from build123d import *

# Parameters (mm, degrees)
REVOLUTION002_ANGLE     = 180
SKETCH015_R             = 1.65
POCKET007_DEPTH         = 7
PAD006_DEPTH            = 3
SKETCH022_R             = 1.65
POCKET012_DEPTH         = 6
BODY004_PLACEMENT_ANGLE = 180


with BuildPart() as part:
    # Sketch014 → Revolution002 (revolve)
    with BuildSketch(Plane.YZ):
        Polygon((-4, 0), (4, 0), (4, 6), (2.5, 6), (0, 4.556624), (-2.5, 6), (-4, 6), align=None)
    revolve(axis=Axis((0, 0, 0), (0, 1, 0)), revolution_arc=REVOLUTION002_ANGLE)

    # Sketch015 → Pocket007 (cut)
    with BuildSketch(Plane(origin=(-5, 0, 0), x_dir=(0, 1, 0), z_dir=(-1, 0, 0))):
        Circle(SKETCH015_R)
    extrude(amount=-POCKET007_DEPTH, mode=Mode.SUBTRACT)

    # Revolution002 Face7 → Pad006 (add)
    with BuildSketch(Plane(origin=(0, 0, 0), x_dir=(0, 1, 0), z_dir=(-1, 0, 0))):
        Polygon((4, -6), (4, 6), (2.5, 6), (0, 4.556624), (-2.5, 6), (-4, 6), (-4, -6), (-2.5, -6), (0, -4.556624), (2.5, -6), align=None)
    extrude(amount=PAD006_DEPTH)

    # Sketch022 (on Face5 of Pad006) → Pocket012 (cut)
    with BuildSketch(Plane(origin=(-3, 0, 0), x_dir=(0, 1, 0), z_dir=(-1, 0, 0))):
        Circle(SKETCH022_R)
    extrude(amount=-POCKET012_DEPTH, mode=Mode.SUBTRACT)


with BuildPart() as part_1:
    # Body004 placement: moved
    add(part.part.moved(Location((11, 0, 19))).rotate(Axis((11, 0, 19), (0, 1, 0)), BODY004_PLACEMENT_ANGLE))


solid = part_1.part
Input: part model. Units: mm. Frame: model coordinates. A direction names the side the tool comes from. Coordinates: 2 decimals unless noted, no trailing zeros. Loops run counter-clockwise (first coordinate to the right, second up) from the corner with the lowest first, then second, coordinate; pieces in that order, holes last.
Q1. Cut plane A-A (y = 1.5). Output: boundary loops of the cut face in (x, z).
Q2. Contact query for a flat-ended pin moving along its axis: pin 1 (1 mm diameter, centred on y = -0.5, z = 19.5, fed in from +X). Output: stop coordinate, or through.
Q3. Set-up query: faces 1 (the face through (6.214, 0.399, 18.895)), 2 (the face through (12.479, 1.233, 13.732)), 3 (the face through (12, 3, 25)), 4 (the face through (8, 0, 19)), 5 (the face through (12.48, 1.27, 24.29)). Return all of +Z, -Z, +X, -X, +Y, -Y with unobstructed straight access to the full face (end or side cutting, diameter ignored); none if empty.
Q4. Draft query along Y for faces 6 (the face through (12, -3, 13)), 7 (the face through (11.042, -0.215, 20.636)), 8 (the face through (10, 4, 19)). Return one class per face: +Y half, -Y half, draft (parallel to the pull), parting line (faces both ways), or undercut.
Q5. Material intervals for line 1 (Z direction, x = 10.5, y = 1); line 2 (Z direction, x = 9.25, y = -0.75); line 3 (Y direction, x = 11.5, z = 24.25), sorted ascending.
Q6. Cut plane B-B (z = 19). Output: boundary loops of the cut face in (x, y).
Working result:
1. outline: (8, 18.31) - (8, 19.69) - (14, 19.69) - (14, 24.42) - (11, 24.42) arc R5.42 ccw to (11, 13.58) - (14, 13.58) - (14, 18.31) - close
2. pin 1: stops at x = 8
3. face 1: -X
3. face 2: -Z, +X, -X
3. face 3: +Z, +X, -X, +Y, -Y
3. face 4: +X
3. face 5: +Z, +X, -X
4. face 6: draft
4. face 7: undercut
4. face 8: +Y half
5. line 1: z = 13.89 to 17.69, 20.31 to 24.11
5. line 2: z = 14.33 to 17.53, 20.47 to 23.67
5. line 3: y = -4 to -1.2, 1.2 to 4
6. outline: (5, -4) - (14, -4) - (14, -1.65) - (8, -1.65) - (8, 1.65) - (14, 1.65) - (14, 4) - (5, 4) - (5, 2.5) - (6.44, 0) - (5, -2.5) - close
